from build123d import *

# Parameters (mm, degrees)
BOSS_EXTRUDE1_DEPTH = 317.5
SKETCH2_W           = 31.75
SKETCH2_H           = 70.720826982
SKETCH2_W_2         = 36.5125
SKETCH2_H_2         = 48.495826983
CUT_EXTRUDE1_DEPTH  = 90.351177502
SKETCH5_W           = 244.475
SKETCH5_H           = 38.1
BOSS_EXTRUDE2_DEPTH = 6.35
CUT_EXTRUDE3_DEPTH  = 97.641296888
FILLET3_R           = 5.08
FILLET4_R           = 3.302


with BuildPart() as part:
    # Sketch1 → Boss-Extrude1 (new body)
    with BuildSketch(Plane(origin=(0, 0, 0), x_dir=(0, 0, -1), z_dir=(1, 0, 0))):
        Polygon((0, 38.1), (-1.238823545, 31.872013469), (-426.688823545, 116.499280171), (-425.45, 122.727266702), align=None)
    extrude(amount=BOSS_EXTRUDE1_DEPTH)

    # Sketch2 → Cut-Extrude1 (cut, through all)
    with BuildSketch(Plane(origin=(0, 36.649905094, -7.290119387), x_dir=(1, 0, 0), z_dir=(0, 0.98078528, -0.195090322))):
        with Locations((15.875, -42.79335476)):
            Rectangle(SKETCH2_W, SKETCH2_H)
        with Locations((18.25625, -416.970086038)):
            Rectangle(SKETCH2_W_2, SKETCH2_H_2)
        with Locations((301.625, -42.79335476)):
            Rectangle(SKETCH2_W, SKETCH2_H)
        with Locations((299.24375, -416.970086038)):
            Rectangle(SKETCH2_W_2, SKETCH2_H_2)
    extrude(amount=-CUT_EXTRUDE1_DEPTH, mode=Mode.SUBTRACT)

    # Sketch5 → Boss-Extrude2 (add)
    with BuildSketch(Plane(origin=(0, 30.421918564, -6.051295842), x_dir=(1, 0, 0), z_dir=(0, -0.98078528, 0.195090322))):
        with Locations((158.75, 460.267999529)):
            Rectangle(SKETCH5_W, SKETCH5_H)
    extrude(amount=-BOSS_EXTRUDE2_DEPTH)

    # Sketch6 → Cut-Extrude3 (cut, through all)
    with BuildSketch(Plane(origin=(0, 30.421918564, -6.051295842), x_dir=(1, 0, 0), z_dir=(0, -0.98078528, 0.195090322))):
        with BuildLine():
            Line((31.75, 26.482941269), (31.75, 7.432941269))
            Line((31.75, 7.432941269), (285.75, 7.432941269))
            Line((285.75, 7.432941269), (285.75, 26.482941269))
            ThreePointArc((285.75, 26.482941269), (158.75, 96.332941269), (31.75, 26.482941269))
        make_face()
    extrude(amount=-CUT_EXTRUDE3_DEPTH, mode=Mode.SUBTRACT)

    # Fillet3
    fillet3_edges = [part.edges().sort_by_distance(p)[0] for p in [
        (285.75, 38.702477369, 19.303371364),
        (31.75, 38.702477369, 19.303371364),
    ]]
    fillet(fillet3_edges, radius=FILLET3_R)

    # Fillet4
    fillet4_edges = [part.edges().sort_by_distance(p)[0] for p in [
        (0, 48.782955644, 69.981357895),
        (0, 110.152206934, 378.505418507),
        (317.5, 110.152206934, 378.505418507),
        (317.5, 48.782955644, 69.981357895),
        (36.5125, 110.152206934, 378.505418507),
        (285.75, 48.782955644, 69.981357895),
        (280.9875, 110.152206934, 378.505418507),
        (31.75, 48.782955644, 69.981357895),
        (36.5125, 127.046214705, 463.437330956),
        (280.9875, 127.046214705, 463.437330956),
    ]]
    fillet(fillet4_edges, radius=FILLET4_R)


solid = part.part
Check sheet for the modelled part. Datum: model origin and axes. Units: mm. A direction names the side the tool comes from. Give positions to 0.01 mm unless a question says otherwise; leave off trailing zeros. Write each loop counter-clockwise with the first axis right and the second up, starting at its lowest first coordinate (ties: lowest second). Pieces come first, ordered by that corner, then holes. Notation, with made-up numbers: (88.25, 9) -> (110.25, 9) arc R10 ccw to (110.25, 15) -> close; hole circle Ø2 at (19.25, 47.5). An arc over 180 degrees is marked (long way). Write item = value, one per line.
Item 1: Gauge pin test, flat ends, axial feed: pin 1 (11 mm diameter, centred on y = 122, z = 440, fed in from +X); pin 2 (6.5 mm diameter, centred on y = 46, z = 59, fed in from +X); pin 3 (11 mm diameter, centred on y = 118.5, z = 438.5, fed in from -X). Record the tip position at first contact, or that the pin passes through.
Output:
pin_1 = 280.99
pin_2 = 285.75
pin_3 = 36.51
Item 2: Sectioned sample at B-B on z = 246.5. Record the boundary of the cut face in (x, y), and give its area (3 significant figures).
Output:
outline = (0, 80.66) -> (317.5, 80.66) -> (317.5, 87.13) -> (0, 87.13) -> close
area = 2,060 mm^2
Item 3: Scan lines: probe 1 along X at (y, z) = (44.5, 64); probe 2 along X at (y, z) = (52.5, 76.5); probe 3 along Y at (x, z) = (162, 363). Record each from-to range of solid material in increasing order. Write a range as from..to.
Output:
probe_1 = 31.75..75.9, 241.6..285.75
probe_2 = 0..102.14, 215.36..317.5
probe_3 = 103.83..110.31
Item 4: Sectioned sample at A-A on x = 20.5. Record the boundary of the cut face in (y, z).
Output:
outline = (45.67, 70.6) -> (51.9, 69.36) -> (113.27, 377.89) -> (107.04, 379.12) -> close
Item 5: Tool access check on faces 1 (the flat face through (36.512, 118, 420)), 2 (the flat face through (285.75, 45, 51)), 3 (the flat face through (31.75, 45, 51)), 4 (the flat face through (280.988, 118, 420)). Record the directions out of +Z, -Z, +X, -X, +Y, -Y that give a thin tool (end or side, any length) a straight path to the whole face; none if there is none.
Output:
face_1 = +Z, -X, +Y, -Y
face_2 = -Z, +X, +Y, -Y
face_3 = -Z, -X, +Y, -Y
face_4 = +Z, +X, +Y, -Y
Item 6: Sectioned sample at C-C on x = 254.5. Record the boundary of the cut face in (y, z).
Output:
outline = (42.5, 54.67) -> (48.73, 53.43) -> (130.16, 462.82) -> (123.93, 464.06) -> close
Item 7: Sectioned sample at D-D on x = 126. Record the boundary of the cut face in (y, z), and give its area (3 significant figures).
Output:
outline = (48.51, 84.89) -> (54.74, 83.65) -> (130.16, 462.82) -> (123.93, 464.06) -> close
area = 2,450 mm^2
